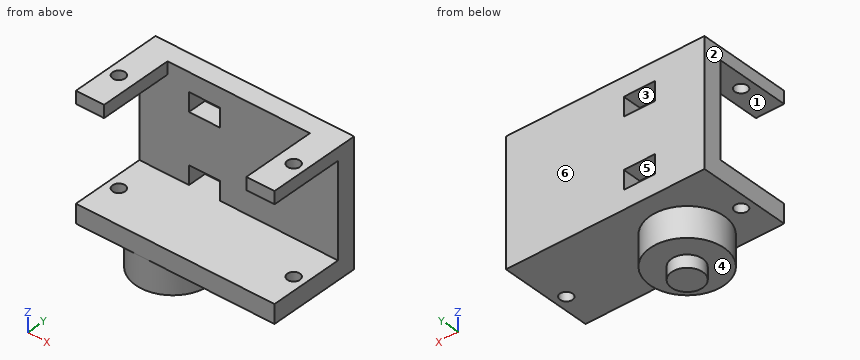
from build123d import *

# Parameters (mm, degrees)
SKETCH1_W            = 31.8
SKETCH1_H            = 13.25
BOSS_EXTRUDE3_DEPTH  = 3
SKETCH3_W            = 31.8
SKETCH3_H            = 3
BOSS_EXTRUDE4_DEPTH  = 24
SKETCH4_W            = 22.8
SKETCH4_H            = 13.25
CUT_EXTRUDE3_DEPTH   = 3
SKETCH6_W            = 31.8
SKETCH6_H            = 2
BOSS_EXTRUDE5_DEPTH  = 13.25
SKETCH7_W            = 3.6
SKETCH7_H            = 3
CUT_EXTRUDE4_DEPTH   = 40.30496947
SKETCH8_W            = 2
SKETCH8_H            = 1.25
BOSS_EXTRUDE6_DEPTH  = 31.8
SKETCH10_W           = 2
SKETCH10_H           = 17.5
CUT_EXTRUDE6_DEPTH   = 38.505207972
BOSS_EXTRUDE7_START  = -31.8
SKETCH11_W           = 3
SKETCH11_H           = 1.25
BOSS_EXTRUDE7_DEPTH  = 31.8
SKETCH12_W           = 22.8
SKETCH12_H           = 1.25
CUT_EXTRUDE7_DEPTH   = 4
SKETCH15_W           = 31.8
SKETCH15_H           = 3
BOSS_EXTRUDE9_DEPTH  = 17.5
BOSS_EXTRUDE12_DEPTH = 5
SKETCH20_W           = 15
SKETCH20_H           = 14.5
SKETCH20_W_2         = 5.230602644
SKETCH20_H_2         = 17.5
CUT_EXTRUDE9_DEPTH   = 100
SKETCH22_R           = 1
SKETCH22_W           = 31.8
SKETCH22_H           = 2.65
CUT_EXTRUDE11_DEPTH  = 20
SKETCH24_R           = 5.925
BOSS_EXTRUDE13_DEPTH = 4.8
SKETCH25_R           = 2.5
BOSS_EXTRUDE14_DEPTH = 2
SKETCH27_W           = 5
SKETCH27_H           = 3
CUT_EXTRUDE12_DEPTH  = 10


with BuildPart() as part:
    # Sketch1 → Boss-Extrude3 (new body)
    with BuildSketch(Plane.XY):
        Rectangle(SKETCH1_W, SKETCH1_H)
    extrude(amount=BOSS_EXTRUDE3_DEPTH)

    # Sketch3 → Boss-Extrude4 (add)
    with BuildSketch(Plane.XY.offset(3)):
        with Locations((0, 8.125)):
            Rectangle(SKETCH3_W, SKETCH3_H)
    extrude(amount=-BOSS_EXTRUDE4_DEPTH)

    # Sketch4 → Cut-Extrude3 (cut)
    with BuildSketch(Plane.XY.offset(3)):
        Rectangle(SKETCH4_W, SKETCH4_H)
    extrude(amount=-CUT_EXTRUDE3_DEPTH, mode=Mode.SUBTRACT)

    # Sketch6 → Boss-Extrude5 (add)
    with BuildSketch(Plane.XZ.offset(-6.625)):
        with Locations((0, -16.4)):
            Rectangle(SKETCH6_W, SKETCH6_H)
    extrude(amount=BOSS_EXTRUDE5_DEPTH)

    # Sketch7 → Cut-Extrude4 (cut, through all)
    with BuildSketch(Plane.ZY.offset(15.9)):
        with Locations((-19.2, 8.125)):
            Rectangle(SKETCH7_W, SKETCH7_H)
    extrude(amount=-CUT_EXTRUDE4_DEPTH, mode=Mode.SUBTRACT)

    # Sketch8 → Boss-Extrude6 (add)
    with BuildSketch(Plane(origin=(15.9, 0, 0), x_dir=(0, 0, -1), z_dir=(1, 0, 0))):
        with Locations((16.4, -7.25)):
            Rectangle(SKETCH8_W, SKETCH8_H)
    extrude(amount=-BOSS_EXTRUDE6_DEPTH)

    # Sketch10 → Cut-Extrude6 (cut, through all)
    with BuildSketch(Plane(origin=(15.9, 0, 0), x_dir=(0, 0, -1), z_dir=(1, 0, 0))):
        with Locations((16.4, 0.875)):
            Rectangle(SKETCH10_W, SKETCH10_H)
    extrude(amount=-CUT_EXTRUDE6_DEPTH, mode=Mode.SUBTRACT)

    # Sketch11 → Boss-Extrude7 (add)
    with BuildSketch(Plane(origin=(15.9, 0, 0), x_dir=(0, 0, -1), z_dir=(1, 0, 0)).offset(BOSS_EXTRUDE7_START)):
        with Locations((-1.5, -7.25)):
            Rectangle(SKETCH11_W, SKETCH11_H)
    boss_extrude7 = extrude(amount=BOSS_EXTRUDE7_DEPTH)

    # Mirror2: Boss-Extrude7 across plane
    add(boss_extrude7.mirror(Plane(origin=(0, 0, 0), x_dir=(0, 0, 1), z_dir=(1, 0, 0))))

    # Sketch12 → Cut-Extrude7 (cut)
    with BuildSketch(Plane.XY.offset(3)):
        with Locations((0, -7.25)):
            Rectangle(SKETCH12_W, SKETCH12_H)
    extrude(amount=-CUT_EXTRUDE7_DEPTH, mode=Mode.SUBTRACT)

    # Sketch15 → Boss-Extrude9 (add)
    with BuildSketch(Plane(origin=(0, 9.625, 0), x_dir=(1, 0, 0), z_dir=(0, 1, 0))):
        with Locations((0, 16.9)):
            Rectangle(SKETCH15_W, SKETCH15_H)
    extrude(amount=-BOSS_EXTRUDE9_DEPTH)

    # Sketch19 → Boss-Extrude12 (add)
    with BuildSketch(Plane.XY.offset(3)):
        Polygon((-15.9, 9.625), (15.9, 9.625), (15.9, -7.875), (11.4, -7.875), (11.4, 6.625), (-11.4, 6.625), (-11.4, -7.875), (-15.9, -7.875), align=None)
    extrude(amount=-BOSS_EXTRUDE12_DEPTH)

    # Sketch20 → Cut-Extrude9 (cut)
    with BuildSketch(Plane.ZY.offset(15.9)):
        with Locations((-7.9, -0.625)):
            Rectangle(SKETCH20_W, SKETCH20_H)
        with Locations((4.215301322, 0.875)):
            Rectangle(SKETCH20_W_2, SKETCH20_H_2)
    extrude(amount=-CUT_EXTRUDE9_DEPTH, mode=Mode.SUBTRACT)

    # Sketch22 → Cut-Extrude11 (cut)
    with BuildSketch(Plane.XY.offset(1.6)):
        with Locations((-14, 0.575)):
            Circle(SKETCH22_R)
        with Locations((14, 0.575)):
            Circle(SKETCH22_R)
        with Locations((0, -6.55)):
            Rectangle(SKETCH22_W, SKETCH22_H)
    extrude(amount=-CUT_EXTRUDE11_DEPTH, mode=Mode.SUBTRACT)

    # Sketch24 → Boss-Extrude13 (add)
    with BuildSketch(Plane(origin=(0, 0, -18.4), x_dir=(-1, 0, 0), z_dir=(0, 0, -1))):
        with Locations(Location((5.47, 0.7, 0), (0, 0, 270))):
            Circle(SKETCH24_R)
    extrude(amount=BOSS_EXTRUDE13_DEPTH)

    # Sketch25 → Boss-Extrude14 (add)
    with BuildSketch(Plane(origin=(0, 0, -23.2), x_dir=(-1, 0, 0), z_dir=(0, 0, -1))):
        with Locations((5.47, 0.7)):
            Circle(SKETCH25_R)
    extrude(amount=BOSS_EXTRUDE14_DEPTH)

    # Sketch27 → Cut-Extrude12 (cut)
    with BuildSketch(Plane.XZ.offset(-6.625)):
        with Locations((-5.47, -13.9)):
            Rectangle(SKETCH27_W, SKETCH27_H)
        with Locations((-5.47, -2.9)):
            Rectangle(SKETCH27_W, SKETCH27_H)
    extrude(amount=-CUT_EXTRUDE12_DEPTH, mode=Mode.SUBTRACT)


solid = part.part
Verification items for the finished model (mm, model axes). Face numbers are marked on the shaded views. A direction names the side the tool comes from. Give positions to 0.01 mm unless a question says otherwise; leave off trailing zeros. Write each loop counter-clockwise with the first axis right and the second up, starting at its lowest first coordinate (ties: lowest second). Pieces come first, ordered by that corner, then holes. Notation, with made-up numbers: M 84.5,20 L 137.5,20 A11 cw 137.5,38 Z; hole C 35.5,86 d10. An arc over 180 degrees is marked long. Use CSV: the item, a comma, the result in double quotes.
1) Access from +Z, -Z, +X, -X, +Y, -Y to the whole of each face (thin tool, end or side, straight path). Record for the marked faces 4, 5 and 6.
Final values:
face 4,"-Z"
face 5,"+Y, -Y"
face 6,"+Z, -Z, +X, -X, +Y"
2) Material ranges on line 1 along Y through (x, z) = (-14, 0.25) (3 decimals); line 2 along X through (y, z) = (-0.25, -16.25); line 3 along Z through (x, y) = (15.5, 9), recorded low to high.
Final values:
line 1,"-5.225 to -0.425, 1.575 to 9.625"
line 2,"-15.9 to -14.57, -13.43 to 13.43, 14.57 to 15.9"
line 3,"-18.4 to 1.6"
3) Go/stop test with flat-tipped pins: pin 1 Ø2 at (x, z) = (3.5, -20.5) entering from -Y; pin 2 Ø4 at (x, y) = (-8, 4) entering from +Z; pin 3 Ø3 at (x, y) = (-1.5, 2.5) entering from -Z; pin 4 Ø2.5 at (x, y) = (-14, 0.575) entering from -Z. Record where each tip stops, or that it passes through.
Final values:
pin 1,"through"
pin 2,"z = -15.4"
pin 3,"z = -23.2"
pin 4,"z = -18.4"
4) Cross-section at D-D (y = -3.25). Enter the section's corners in (x, z), plus the area to 3 significant figures.
Final values:
outline,"M -15.9,-18.4 L -9.89,-18.4 L -9.89,-23.2 L -1.05,-23.2 L -1.05,-18.4 L 15.9,-18.4 L 15.9,-15.4 L -15.9,-15.4 Z; M -15.9,-0.4 L -11.4,-0.4 L -11.4,1.6 L -15.9,1.6 Z; M 11.4,-0.4 L 15.9,-0.4 L 15.9,1.6 L 11.4,1.6 Z"
area,"156 mm²"
5) Release check for a two-part mould opening along X. For the marked faces 1, 2 and 3 record: released by +X, released by -X, zero draft, split by the parting line, or undercut.
Final values:
face 1,"zero draft"
face 2,"released by -X"
face 3,"undercut"
6) Cross-section at B-B (y = 7.75). Enter the section's corners in (x, z), plus the area to 3 significant figures.
Final values:
outline,"M -15.9,-18.4 L 15.9,-18.4 L 15.9,1.6 L -15.9,1.6 Z; hole M -7.97,-15.4 L -2.97,-15.4 L -2.97,-12.4 L -7.97,-12.4 Z; hole M -7.97,-4.4 L -2.97,-4.4 L -2.97,-1.4 L -7.97,-1.4 Z"
area,"606 mm²"
7) Cross-section at C-C (x = 14). Enter the section's corners in (y, z) (3 decimals).
Final values:
outline,"M -5.225,-18.4 L -0.425,-18.4 L -0.425,-15.4 L -5.225,-15.4 Z; M -5.225,-0.4 L -0.425,-0.4 L -0.425,1.6 L -5.225,1.6 Z; M 1.575,-18.4 L 9.625,-18.4 L 9.625,1.6 L 1.575,1.6 L 1.575,-0.4 L 6.625,-0.4 L 6.625,-15.4 L 1.575,-15.4 Z"
8) Cross-section at A-A (z = -14). Enter the section's corners in (x, y) (3 decimals).
Final values:
outline,"M -15.9,6.625 L -7.97,6.625 L -7.97,9.625 L -15.9,9.625 Z; M -2.97,6.625 L 15.9,6.625 L 15.9,9.625 L -2.97,9.625 Z"
